The listing builds one solid part. Answer for the finished solid, in the listing's coordinates (mm). A direction names the side the tool comes from. Round coordinates to 2 decimals unless told otherwise and drop trailing zeros. Loops run counter-clockwise (first coordinate to the right, second up) from the corner with the lowest first, then second, coordinate; pieces in that order, holes last. Notation, with made-up numbers: (-5, 23.5) - (40, 23.5) arc R17 ccw to (40, 45.5) - close; hole circle Ø8 at (20.25, 29). An arc over 180 degrees is marked (long way). One line per item, written item: value.
```python
from build123d import *

# Parameters (mm, degrees)
BOSS_EXTRUDE1_DEPTH = 12.7
FILLET1_R           = 3
FILLET2_R           = 20
CUT_EXTRUDE1_REACH  = 88.899
SKETCH2_R           = 2.3
SKETCH2_3_R         = 4.5
SKETCH2_3_R_2       = 2.3
CUT_EXTRUDE2_DEPTH  = 2
FILLET3_R           = 1
FILLET4_R           = 1


with BuildPart() as part:
    # Sketch1 → Boss-Extrude1 (new body)
    with BuildSketch(Plane.XY):
        with BuildLine():
            Line((-60.8, 0), (-60.8, 80))
            Line((-60.8, 80), (-73.5, 80))
            Line((-73.5, 80), (-73.5, 0))
            ThreePointArc((-73.5, 0), (-66.0323905, -32.279612836), (-45.14698218, -58))
            Line((-45.14698218, -58), (-18.238420984, -58))
            ThreePointArc((-18.238420984, -58), (-49.018037475, -35.970432331), (-60.8, 0))
        make_face()
    extrude(amount=BOSS_EXTRUDE1_DEPTH)

    # Fillet1
    fillet1_edges = [part.edges().sort_by_distance(p)[0] for p in [
        (-18.238420984, -58, 6.35),
    ]]
    fillet(fillet1_edges, radius=FILLET1_R)

    # Fillet2
    fillet2_edges = [part.edges().sort_by_distance(p)[0] for p in [
        (-45.14698218, -58, 6.35),
    ]]
    fillet(fillet2_edges, radius=FILLET2_R)

    # Sketch2 → Cut-Extrude1 (cut, up to next)
    with BuildSketch(Plane(origin=(-60.8, 0, 0), x_dir=(0, 0, -1), z_dir=(1, 0, 0)), mode=Mode.PRIVATE) as cut_extrude1_sk1:
        with Locations((-6.35, 34.28)):
            Circle(SKETCH2_R)
    cut_extrude1_tool1 = extrude(cut_extrude1_sk1.sketch, amount=-CUT_EXTRUDE1_REACH, mode=Mode.PRIVATE) & part.part
    # Sketch2 → Cut-Extrude1 (cut, up to next)
    with BuildSketch(Plane(origin=(-60.8, 0, 0), x_dir=(0, 0, -1), z_dir=(1, 0, 0)), mode=Mode.PRIVATE) as cut_extrude1_sk2:
        with Locations((-6.35, 21.58)):
            Circle(SKETCH2_R)
    cut_extrude1_tool2 = extrude(cut_extrude1_sk2.sketch, amount=-CUT_EXTRUDE1_REACH, mode=Mode.PRIVATE) & part.part
    add(cut_extrude1_tool1.solids().sort_by_distance((-60.8, 34.28, 6.35))[0], mode=Mode.SUBTRACT)
    add(cut_extrude1_tool2.solids().sort_by_distance((-60.8, 21.58, 6.35))[0], mode=Mode.SUBTRACT)

    # Sketch2_3 → Cut-Extrude2 (cut)
    # profile 1 of 2: a face of its own
    with BuildSketch(Plane(origin=(-60.8, 0, 0), x_dir=(0, 0, -1), z_dir=(1, 0, 0))):
        with Locations((-6.35, 34.28)):
            Circle(SKETCH2_3_R)
        with Locations((-6.35, 34.28)):
            Circle(SKETCH2_3_R_2, mode=Mode.SUBTRACT)
    # profile 2 of 2: a face of its own
    with BuildSketch(Plane(origin=(-60.8, 0, 0), x_dir=(0, 0, -1), z_dir=(1, 0, 0))):
        with Locations((-6.35, 21.58)):
            Circle(SKETCH2_3_R)
        with Locations((-6.35, 21.58)):
            Circle(SKETCH2_3_R_2, mode=Mode.SUBTRACT)
    extrude(amount=-CUT_EXTRUDE2_DEPTH, mode=Mode.SUBTRACT)

    # Fillet3
    fillet3_edges = [part.edges().sort_by_distance(p)[0] for p in [
        (-73.5, 40, 12.7),
        (-52.773401506, -30.192848383, 0),
        (-52.773401506, -30.192848383, 12.7),
        (-29.438560761, -55.787838597, 0),
        (-67.841711996, -28.279888852, 12.7),
        (-29.438560761, -55.787838597, 12.7),
        (-34.99646236, -58, 0),
        (-34.99646236, -58, 12.7),
        (-45.271750842, -56.494758035, 0),
        (-45.271750842, -56.494758035, 12.7),
        (-67.841711996, -28.279888852, 0),
        (-73.5, 40, 0),
        (-60.8, 40, 0),
        (-60.8, 40, 12.7),
    ]]
    fillet(fillet3_edges, radius=FILLET3_R)

    # Fillet4
    fillet4_edges = [part.edges().sort_by_distance(p)[0] for p in [
        (-73.5, 80, 6.35),
        (-67.15, 80, 0),
        (-67.15, 80, 12.7),
        (-60.8, 80, 6.35),
        (-61.092893219, 80, 12.407106781),
        (-61.092893219, 80, 0.292893219),
        (-73.207106781, 80, 12.407106781),
        (-73.207106781, 80, 0.292893219),
    ]]
    fillet(fillet4_edges, radius=FILLET4_R)


solid = part.part
```
1) Consider L1, parallel to Z at x = -70, y = 34; L2, parallel to Y at x = -68, z = 6.35; L3, parallel to Y at x = -61.45, z = 6.35. Determine where each line is inside the solid, lowest interval first.
Final values:
L1: 0 to 4.07, 8.63 to 12.7
L2: -27.9 to 19.28, 23.88 to 31.98, 36.58 to 80
L3: -40.33 to 17.08, 26.08 to 29.78, 38.78 to 79.94
2) A cutting plane is placed at B-B on z = 6.35. Give the vertices of the cut face in (x, y).
Final values:
outline: (-73.5, 0) arc R73.5 ccw to (-51.74, -52.21) arc R20 ccw to (-37.66, -58) - (-32.33, -58) arc R3 ccw to (-30.81, -52.41) arc R60.8 cw to (-60.8, 0) - (-60.8, 17.08) - (-62.8, 17.08) - (-62.8, 19.28) - (-73.5, 19.28) - close; (-73.5, 23.88) - (-62.8, 23.88) - (-62.8, 26.08) - (-60.8, 26.08) - (-60.8, 29.78) - (-62.8, 29.78) - (-62.8, 31.98) - (-73.5, 31.98) - close; (-73.5, 36.58) - (-62.8, 36.58) - (-62.8, 38.78) - (-60.8, 38.78) - (-60.8, 79) arc R1 ccw to (-61.8, 80) - (-72.5, 80) arc R1 ccw to (-73.5, 79) - close
3) Each of these flat-tipped pins is pushed along its axis until it touches: pin 1 Ø4 at (y, z) = (34.28, 6.35) entering from -X; pin 2 Ø5.5 at (y, z) = (21.58, 6.35) entering from +X; pin 3 Ø1.5 at (x, z) = (-37.5, 2.5) entering from +Y; pin 4 Ø1 at (y, z) = (57.5, 5) entering from +X. Where does it stop, or does it pass through?
Final values:
pin 1: through
pin 2: x = -62.8
pin 3: y = -47.26
pin 4: x = -60.8
4) A cutting plane is placed at A-A on y = 21.58. Give the vertices of the cut face in (x, z).
Final values:
outline: (-73.5, 1) arc R1 ccw to (-72.5, 0) - (-61.8, 0) arc R1 ccw to (-60.8, 1) - (-60.8, 1.85) - (-62.8, 1.85) - (-62.8, 4.05) - (-73.5, 4.05) - close; (-73.5, 8.65) - (-62.8, 8.65) - (-62.8, 10.85) - (-60.8, 10.85) - (-60.8, 11.7) arc R1 ccw to (-61.8, 12.7) - (-72.5, 12.7) arc R1 ccw to (-73.5, 11.7) - close
5) For faces 1 (the cylindrical face through (-61.79, 38.74, 6.94)), 2 (the flat face through (-73.5, 40, 6)), 3 (the flat face through (-60.8, 39, 6)), determine the directions among +Z, -Z, +X, -X, +Y, -Y from which every point of the face is accessible in a straight line to the end or side of a thin tool.
Final values:
face 1: +X
face 2: +Z, -Z, -X, +Y, -Y
face 3: +Z, -Z, +X, +Y
